Autodesk Inventor part; units mm, degrees
ref_plane "YZ Plane" through (0, 0, 0) normal (1, 0, 0) x (0, 1, 0)
ref_plane "XZ Plane" through (0, 0, 0) normal (0, 1, 0) x (-1, 0, 0)
ref_plane "XY Plane" through (0, 0, 0) normal (0, 0, 1) x (1, 0, 0)
sketch "Sketch1" plane through (0, 0, 0) normal (0, 1, 0) x (-1, 0, 0)
  line L0 (-85, 85) -> (85, 85)
  line L1 (85, 85) -> (85, -85)
  line L2 (85, -85) -> (-85, -85)
  line L3 (-85, -85) -> (-85, 85)
  line L4 (-85, 85) -> (85, -85) construction
  line L5 (85, 85) -> (-85, -85) construction
  point P0 (0, 0)
  point P1 (-63, -63)
  point P2 (-63, -21)
  point P3 (-63, 21)
  point P4 (-63, 63)
  point P5 (-21, -63)
  point P6 (-21, -21)
  point P7 (-21, 21)
  point P8 (-21, 63)
  point P9 (21, -63)
  point P10 (21, -21)
  point P11 (21, 21)
  point P12 (21, 63)
  point P13 (63, -63)
  point P14 (63, -21)
  point P15 (63, 21)
  point P16 (63, 63)
  dimension "d0" = 170
  dimension "d1" = 170
  dimension "d4" = 42
  dimension "d7" = 42
extrude "Extrusion1" add sketch "Sketch1" along normal blind 9
hole "Hole1" at (63, 0, -63) at (63, 0, -21) at (63, 0, 21) at (63, 0, 63) at (21, 0, -63) at (21, 0, -21) at (21, 0, 21) at (21, 0, 63) at (-21, 0, -63) at (-21, 0, -21) at (-21, 0, 21) at (-21, 0, 63) at (-63, 0, -63) at (-63, 0, -21) at (-63, 0, 21) at (-63, 0, 63) direction (0, 1, 0) diameter 21 end through all both
sketch "Sketch2" plane through (0, 9, 0) normal (0, 1, 0) x (1, 0, 0)
  line L0 (-33.7, -4.15) -> (33.7, -4.15)
  line L1 (33.7, -4.15) -> (33.7, 4.15)
  line L2 (33.7, 4.15) -> (-33.7, 4.15)
  line L3 (-33.7, 4.15) -> (-33.7, -4.15)
  line L4 (-33.7, -4.15) -> (33.7, 4.15) construction
  line L5 (33.7, -4.15) -> (-33.7, 4.15) construction
  point P0 (0, 0)
  dimension "d19" = 67.4
  dimension "d20" = 8.3
sketch "Sketch3" plane through (0, 9, 0) normal (0, 1, 0) x (1, 0, 0)
  line L0 (-42.7949, -50) -> (42.7949, -50) construction
  line L1 (42.7949, -50) -> (42.7949, 50) construction
  line L2 (42.7949, 50) -> (-42.7949, 50) construction
  line L3 (-42.7949, 50) -> (-42.7949, -50) construction
  line L4 (-42.7949, -50) -> (42.7949, 50) construction
  line L5 (42.7949, -50) -> (-42.7949, 50) construction
  point P0 (25, -42.5)
  point P1 (0, 0)
  dimension "d31" = 100
hole "Hole3" at (-42.7949, 9, -50) at (42.7949, 9, -50) at (42.7949, 9, 50) at (-42.7949, 9, 50) direction (0, -1, 0) diameter 6 end through all both
sketch "Sketch4" plane through (0, 9, 0) normal (0, 1, 0) x (1, 0, 0)
  circle A0 centre (42.7949, -50) radius 3 construction
  circle A1 centre (-42.7949, 50) radius 3 construction
  circle A2 centre (42.7949, 50) radius 3 construction
  circle A3 centre (-42.7949, -50) radius 3 construction
  circle A4 centre (-63, -21) radius 10.5 construction
  circle A5 centre (-63, 63) radius 10.5 construction
  circle A6 centre (-21, -21) radius 10.5 construction
  circle A7 centre (-21, 63) radius 10.5 construction
  circle A8 centre (21, -21) radius 10.5 construction
  circle A9 centre (21, 63) radius 10.5 construction
  circle A10 centre (63, -21) radius 10.5 construction
  circle A11 centre (63, 63) radius 10.5 construction
  circle A12 centre (63, 21) radius 10.5 construction
  circle A13 centre (63, -63) radius 10.5 construction
  circle A14 centre (21, 21) radius 10.5 construction
  circle A15 centre (21, -63) radius 10.5 construction
  circle A16 centre (-21, 21) radius 10.5 construction
  circle A17 centre (-21, -63) radius 10.5 construction
  circle A18 centre (-63, 21) radius 10.5 construction
  circle A19 centre (-63, -63) radius 10.5 construction
  line L0 (-85, -85) -> (85, -85) construction
  line L1 (85, -85) -> (85, 85) construction
  line L2 (85, 85) -> (-85, 85) construction
  line L3 (-85, 85) -> (-85, -85) construction
  line L4 (-85, 85) -> (85, 85) construction
  line L5 (-7.5, -85) -> (7.5, -85) construction
  line L6 (7.5, -85) -> (7.5, 85) construction
  line L7 (7.5, 85) -> (-7.5, 85) construction
  line L8 (-7.5, 85) -> (-7.5, -85) construction
  line L9 (-7.5, -85) -> (7.5, 85) construction
  line L10 (7.5, -85) -> (-7.5, 85) construction
  line L11 (-21, 63) -> (21, 63) construction
  line L12 (21, 63) -> (21, 21) construction
  line L13 (21, 21) -> (-21, 21) construction
  line L14 (-21, 21) -> (-21, 63) construction
  line L15 (-85, 0) -> (85, 0) construction
  point P0 (0, 0)
  point P1 (0, 42)
  point P2 (0, -42)
  dimension "d39" = 15
hole "Hole4" at (0, 9, -42) at (0, 9, 42) direction (0, -1, 0) diameter 6 end through all both
sketch "Sketch5" plane through (0, 9, 0) normal (0, 1, 0) x (1, 0, 0)
  line L0 (-33.7, -7.5) -> (33.7, -7.5) construction
  line L1 (33.7, -7.5) -> (33.7, 7.5) construction
  line L2 (33.7, 7.5) -> (-33.7, 7.5) construction
  line L3 (-33.7, 7.5) -> (-33.7, -7.5) construction
  line L4 (-33.7, -7.5) -> (33.7, 7.5) construction
  line L5 (33.7, -7.5) -> (-33.7, 7.5) construction
  line L6 (0, 7.5) -> (0, -7.5) construction
  line L7 (-1.8038, 7.5) -> (0, 4.1128)
  line L8 (1.8038, 7.5) -> (0, 4.1128)
  line L9 (-1.8038, 7.5) -> (1.8038, 7.5)
  line L10 (-33.7, 0) -> (33.7, 0) construction
  line L11 (-1.8038, -7.5) -> (0, -4.1128)
  line L12 (1.8038, -7.5) -> (0, -4.1128)
  line L13 (-1.8038, -7.5) -> (1.8038, -7.5)
  line L14 (-16.8038, 7.5) -> (-15, 4.1128)
  line L15 (-13.1962, 7.5) -> (-15, 4.1128)
  line L16 (-16.8038, 7.5) -> (-13.1962, 7.5)
  line L17 (13.1962, 7.5) -> (15, 4.1128)
  line L18 (16.8038, 7.5) -> (15, 4.1128)
  line L19 (13.1962, 7.5) -> (16.8038, 7.5)
  line L20 (-1.8038, 7.5) -> (0, 4.1128)
  line L21 (1.8038, 7.5) -> (0, 4.1128)
  line L22 (-1.8038, 7.5) -> (1.8038, 7.5)
  line L23 (-16.8038, -7.5) -> (-15, -4.1128)
  line L24 (-13.1962, -7.5) -> (-15, -4.1128)
  line L25 (-16.8038, -7.5) -> (-13.1962, -7.5)
  line L26 (13.1962, -7.5) -> (15, -4.1128)
  line L27 (16.8038, -7.5) -> (15, -4.1128)
  line L28 (13.1962, -7.5) -> (16.8038, -7.5)
  point P0 (0, 0)
  point P1 (-15, 7.5)
  point P2 (15, 7.5)
  point P3 (-15, -7.5)
  point P4 (15, -7.5)
  dimension "d47" = 67.4
  dimension "d50" = 15
  dimension "d53" = 15
  dimension "d56" = 15
extrude "Extrusion2" cut sketch "Sketch5" against normal blind 10 contours L9 L8 L7 | L11 L12 L13
extrude "Extrusion3" cut sketch "Sketch5" against normal blind 10 contours L16 L15 L14 | L19 L18 L17 | L23 L24 L25 | L26 L27 L28
properties part number "back_plate"
Work out the finished part from the listing and answer in its coordinate system (mm). Give positions to 0.01 mm unless a question says otherwise; leave off trailing zeros. Loops run counter-clockwise (first coordinate to the right, second up) from the corner with the lowest first, then second, coordinate; pieces in that order, holes last. Notation, with made-up numbers: (-18.5, 65.25) -> (29.5, 65.25) arc R17 cw to (29.5, 86.25) -> close; hole circle Ø11 at (65, -25). An arc over 180 degrees is marked (long way). Use CSV: the item, a comma, the result in double quotes.
1. The part is cut by section C-C (z = -63). Write down the section's boundary in (x, y).
Found:
outline,"(-85, 0) -> (-73.5, 0) -> (-73.5, 9) -> (-85, 9) -> close; (-52.5, 0) -> (-31.5, 0) -> (-31.5, 9) -> (-52.5, 9) -> close; (-10.5, 0) -> (10.5, 0) -> (10.5, 9) -> (-10.5, 9) -> close; (31.5, 0) -> (52.5, 0) -> (52.5, 9) -> (31.5, 9) -> close; (73.5, 0) -> (85, 0) -> (85, 9) -> (73.5, 9) -> close"
2. Straight lines are drawn through the part: line 1 (Z direction, x = -21, y = 7); line 2 (Z direction, x = -42.5, y = 4.5). For each, find the intervals that lie inside material, in ascending order.
Found:
line 1,"-85 to -73.5, -52.5 to -31.5, -10.5 to 10.5, 31.5 to 52.5, 73.5 to 85"
line 2,"-85 to -52.99, -47.01 to 47.01, 52.99 to 85"
3. The part is cut by section B-B (z = 42). Write down the section's boundary in (x, y), then the cut area to 3 significant figures.
Found:
outline,"(-85, 0) -> (-3, 0) -> (-3, 9) -> (-85, 9) -> close; (3, 0) -> (85, 0) -> (85, 9) -> (3, 9) -> close"
area,"1,480 mm^2"
4. The mould has two halves that part along Z. Classify faces 1 (the flat face through (1, 0, 1)), 2 (the flat face through (-1, 4, -85)), 3 (the cylindrical face through (69.39, 4.56, 71.33)): +Z half, -Z half, draft (parallel to the pull), parting line (faces both ways), or undercut.
Found:
face 1,"draft"
face 2,"-Z half"
face 3,"undercut"
5. The part is cut by section D-D (y = 7.25). State how many separate pieces and enclosed holes the cut face has, then the cut area to 3 significant figures.
Found:
separate pieces,"1"
enclosed holes,"28"
area,"23,200 mm^2"
6. The part is cut by section A-A (x = 63). Write down the section's boundary in (y, z), then the cut area to 3 significant figures.
Found:
outline,"(0, -85) -> (9, -85) -> (9, -73.5) -> (0, -73.5) -> close; (0, -52.5) -> (9, -52.5) -> (9, -31.5) -> (0, -31.5) -> close; (0, -10.5) -> (9, -10.5) -> (9, 10.5) -> (0, 10.5) -> close; (0, 31.5) -> (9, 31.5) -> (9, 52.5) -> (0, 52.5) -> close; (0, 73.5) -> (9, 73.5) -> (9, 85) -> (0, 85) -> close"
area,"774 mm^2"
